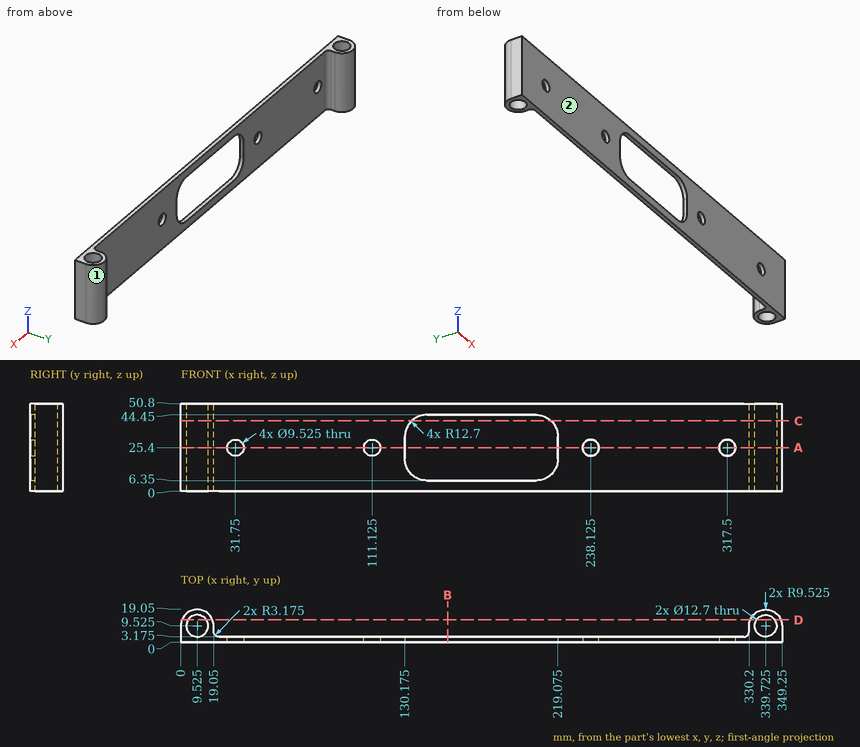
The drawing under review shows one solid part. Ordinate dimensions are in mm from its lowest x, y, z. Coordinates: 2 decimals unless noted, no trailing zeros. Order: outer loops, then holes, each group sorted by start corner. A loop starts at its lowest first (then second) coordinate and runs counter-clockwise, first axis right, second up. Notation, with made-up numbers: (-30.75, -14.75) -> (3.25, -14.75) arc R14 ccw to (3.25, -4.75) -> close; hole circle Ø10 at (-32.5, 29.5). An arc over 180 degrees is marked (long way). One line per item, written item: value.
1) To check wall thickness, follow probe 1 along X at (y, z) = (10.25, 33); probe 2 along X at (y, z) = (11.75, 29); probe 3 along Z at (x, y) = (317.5, 2.55). State the ranges of each line that lie inside material, in increasing order. Write a range as [from, to].
Output values:
probe 1: x = [0.03, 3.22], [15.83, 19.02], [330.23, 333.42], [346.03, 349.22]
probe 2: x = [0.26, 3.58], [15.47, 18.79], [330.46, 333.78], [345.67, 348.99]
probe 3: z = [0, 20.64], [30.16, 50.8]
2) We need section B-B, the plane x = 155. Give the boundary of the cut face in (y, z) (3 decimals).
Output values:
outline: (0, 0) -> (3.175, 0) -> (3.175, 6.35) -> (0, 6.35) -> close; (0, 44.45) -> (3.175, 44.45) -> (3.175, 50.8) -> (0, 50.8) -> close
3) We need section A-A, the plane z = 25.4. Count the separate pieces of the cut face and the enclosed holes in it, then the cut area to 3 significant figures.
Output values:
separate pieces: 6
enclosed holes: 2
area: 984 mm2
4) Draft analysis for pull direction Y (two halves, no side actions). For the marked faces 1 and 2, state which applies: +Y half, -Y half, draft (parallel to the pull), parting line (faces both ways), or undercut.
Output values:
face 1: +Y half
face 2: -Y half
5) We need section D-D, the plane y = 13. Give the boundary of the cut face in (x, z).
Output values:
outline: (0.66, 0) -> (4.21, 0) -> (4.21, 50.8) -> (0.66, 50.8) -> close; (14.84, 0) -> (18.39, 0) -> (18.39, 50.8) -> (14.84, 50.8) -> close; (330.86, 0) -> (334.41, 0) -> (334.41, 50.8) -> (330.86, 50.8) -> close; (345.04, 0) -> (348.59, 0) -> (348.59, 50.8) -> (345.04, 50.8) -> close
6) Clearance check with flat-ended pins moving along their axes: P1, Ø2, axis at y = 12.5, z = 42, coming from the +X side; P2, Ø12.5, axis at x = 317.5, z = 25.4, coming from the +Y side (3 decimals). State where each tip first meets the part, or that it passes through.
Output values:
P1: stops at x = 349.04
P2: stops at y = 3.175
7) We need section C-C, the plane z = 41. Give the boundary of the cut face in (x, y) (3 decimals).
Output values:
outline: (0, 0) -> (134.173, 0) -> (134.173, 3.175) -> (22.225, 3.175) arc R3.175 cw to (19.05, 6.35) -> (19.05, 9.525) arc R9.525 ccw to (0, 9.525) -> close; (215.077, 0) -> (349.25, 0) -> (349.25, 9.525) arc R9.525 ccw to (330.2, 9.525) -> (330.2, 6.35) arc R3.175 cw to (327.025, 3.175) -> (215.077, 3.175) -> close; hole circle Ø12.7 at (9.525, 9.525); hole circle Ø12.7 at (339.725, 9.525)
